Verification items for this drawing (mm, ordinates from the low corner). Give positions to 0.01 mm unless a question says otherwise; leave off trailing zeros. Loops run counter-clockwise (first coordinate to the right, second up) from the corner with the lowest first, then second, coordinate; pieces in that order, holes last. Notation, with made-up numbers: (50, 21) -> (64, 21) arc R25 ccw to (64, 51) -> close; hole circle Ø6 at (-14, 73). An arc over 180 degrees is marked (long way). Write each question's results on one line, items separated by ' | '. Start each with the question number.
Item 1: Cross-section at A-A on x = 90. Enter the section's corners in (y, z).
Item 2: Cross-section at C-C on z = 13. Enter the section's corners in (x, y), then the cut area to 3 significant figures.
Item 3: Mould release check, pull along Y, two halves, no side actions. Record for the marked faces 1, 2 and 3: pulls with the +Y half, pulls with the -Y half, needs draft (parallel to the pull), parting line crosses it, or undercut.
Item 4: Gauge pin test, flat ends, axial feed: pin 1 Ø17 at (x, z) = (93.61, 96.25) entering from -Y; pin 2 Ø5 at (x, y) = (29, 3.5) entering from +Z (1 decimal); pin 3 Ø1 at (x, y) = (156, 7.5) entering from -Z (1 decimal); pin 4 Ø8 at (x, z) = (82.79, 90) entering from +Y. Record the tip position at first contact, or that the pin passes through.
Item 5: Cross-section at D-D on x = 122.5. Enter the section's corners in (y, z).
Item 6: Scan lines: line 1 along Z through (x, y) = (96.5, 14) (1 decimal); line 2 along Z through (x, y) = (151, 13.5) (1 decimal); line 3 along Z through (x, y) = (78, 11) (1 decimal). Record each from-to range of solid material in increasing order.
Item 7: Cross-section at B-B on y = 2.5. Enter the section's corners in (x, z), then the cut area to 3 significant figures.
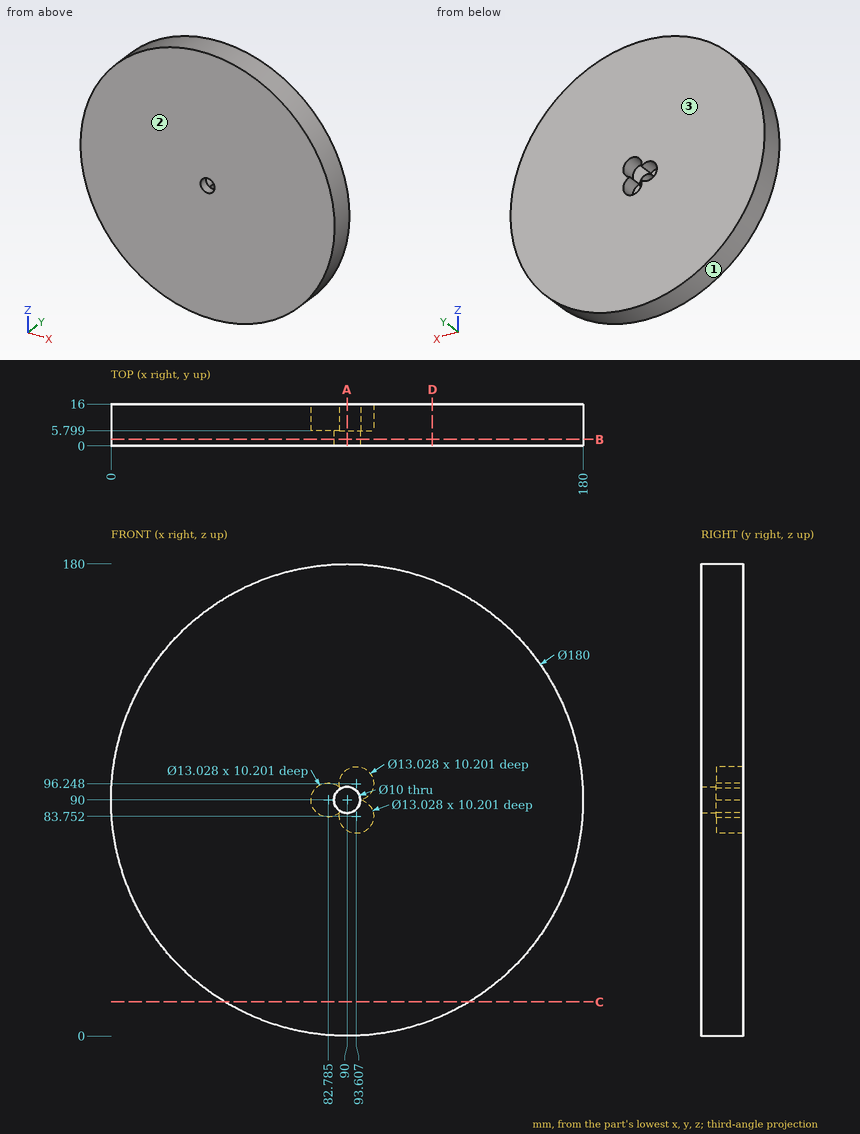
Answer sheet:
1) outline: (0, 0) -> (16, 0) -> (16, 78.33) -> (5.8, 78.33) -> (5.8, 85) -> (0, 85) -> close; (0, 95) -> (5.8, 95) -> (5.8, 101.67) -> (16, 101.67) -> (16, 180) -> (0, 180) -> close
2) outline: (43.41, 0) -> (136.59, 0) -> (136.59, 16) -> (43.41, 16) -> close | area: 1,490 mm²
3) face 1: needs draft | face 2: pulls with the -Y half | face 3: pulls with the +Y half
4) pin 1: stops at y = 0 | pin 2: stops at z = 158.4 | pin 3: stops at z = 28.3 | pin 4: stops at y = 5.8
5) outline: (0, 6.07) -> (16, 6.07) -> (16, 173.93) -> (0, 173.93) -> close
6) line 1: z = 0.2 to 77.9, 89.6 to 90.4, 102.1 to 179.8 | line 2: z = 23.8 to 156.2 | line 3: z = 0.8 to 85.6, 94.4 to 179.2
7) outline: circle Ø180 at (90, 90); hole circle Ø10 at (90, 90) | area: 25,400 mm²
